Could you check a few things on this drawing? It's one solid part, dimensions in mm from its lowest x, y, z. A direction names the side the tool comes from. Give positions to 0.01 mm unless a question says otherwise; leave off trailing zeros. Loops run counter-clockwise (first coordinate to the right, second up) from the corner with the lowest first, then second, coordinate; pieces in that order, holes last. Notation, with made-up numbers: (66, 15.5) - (100, 15.5) arc R22 cw to (100, 41.5) - close; hole circle Ø1 at (-5, -11). An arc over 180 degrees is marked (long way). Return JSON: item names as keys, results as strings. Group by question number.
(1) I need wall thicknesses on probe 1 along X at (y, z) = (37.5, 27.5); probe 2 along Y at (x, z) = (89, 44.5); probe 3 along Z at (x, y) = (56, 85). Which ranges of each line are inside material? Lowest first, please. Write a range as [from, to].
(2) If we section it at D-D (y = 59): Please give me the cut outline in (x, z).
(3) If we section it at A-A (x = 30): Please give me the cut outline in (y, z).
(4) If we section it at B-B (y = 24): Please give me the cut outline in (x, z).
(5) If we section it at C-C (z = 30): Please give me the cut outline in (x, y), then the cut area to 3 significant figures.
(6) On a 3-axis mill with a long thin cutter (end or side, diameter ignored), from which of +Z, -Z, +X, -X, +Y, -Y can I reach the whole of each face in a straight line? I mean the marked faces 1 and 2. Say none if no direction works.
(7) For P1, Ø6, axis at x = 45.5, y = 11, coming from the -Z side; P2, Ø1.8, axis at x = 2.5, z = 9, coming from the +Y side; P3, Ø3, axis at x = 1, z = 16.5, coming from the -Y side, each with a flat end and sliding along its axis, tell me the tip position at first contact or that it passes through.
(8) If we mould it in two halves opening along X, with no side actions, what happens to the marked faces 3, 4 and 5? For each: released by +X, released by -X, zero draft, split by the parting line, or undercut.
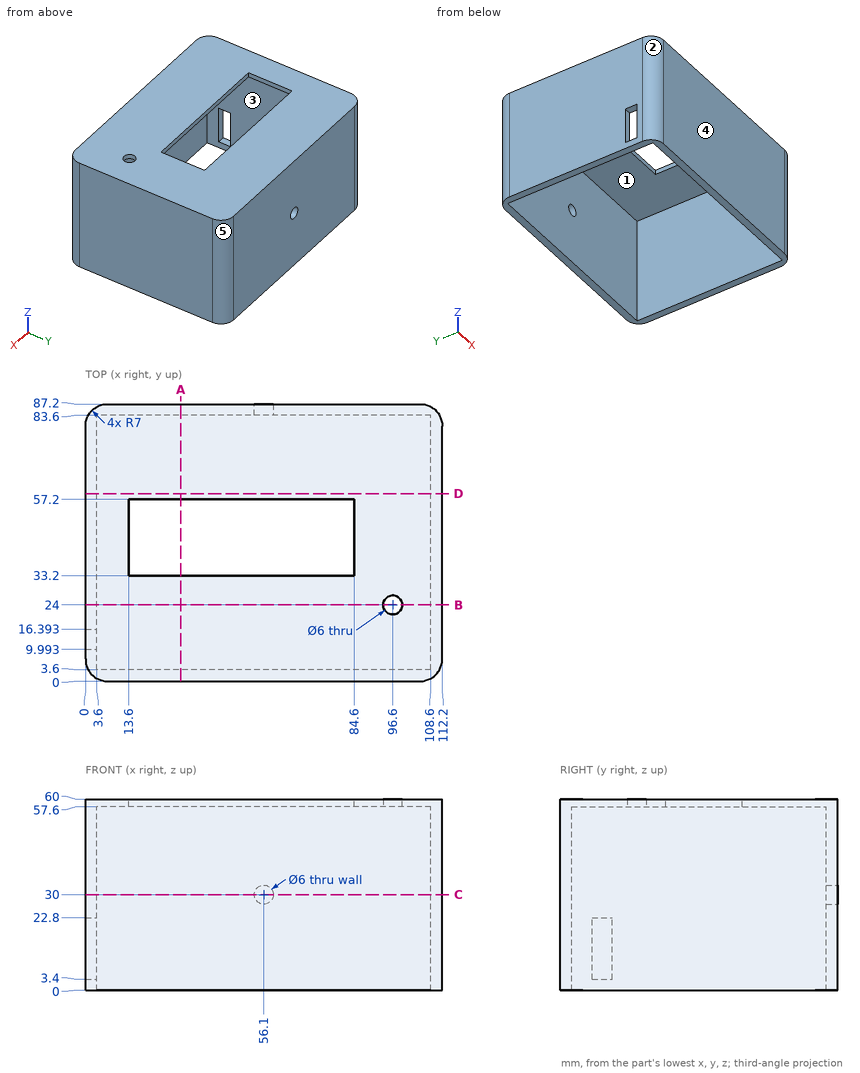
Values:
{
 "1": {"probe 1": "[0, 3.6], [108.6, 112.2]", "probe 2": "[0, 3.6], [83.6, 87.2]", "probe 3": "[0, 27], [33, 60]"},
 "2": {"outline": "(0, 0) - (3.6, 0) - (3.6, 57.6) - (108.6, 57.6) - (108.6, 0) - (112.2, 0) - (112.2, 60) - (0, 60) - close"},
 "3": {"outline": "(0, 0) - (3.6, 0) - (3.6, 57.6) - (33.2, 57.6) - (33.2, 60) - (0, 60) - close; (57.2, 57.6) - (83.6, 57.6) - (83.6, 0) - (87.2, 0) - (87.2, 60) - (57.2, 60) - close"},
 "4": {"outline": "(0, 0) - (3.6, 0) - (3.6, 57.6) - (93.6, 57.6) - (93.6, 60) - (0, 60) - close; (99.6, 57.6) - (108.6, 57.6) - (108.6, 0) - (112.2, 0) - (112.2, 60) - (99.6, 60) - close"},
 "5": {"outline": "(0, 7) arc R7 ccw to (7, 0) - (105.2, 0) arc R7 ccw to (112.2, 7) - (112.2, 80.2) arc R7 ccw to (105.2, 87.2) - (59.1, 87.2) - (59.1, 83.6) - (108.6, 83.6) - (108.6, 3.6) - (3.6, 3.6) - (3.6, 83.6) - (53.1, 83.6) - (53.1, 87.2) - (7, 87.2) arc R7 ccw to (0, 80.2) - close", "area": "1,320 mm2"},
 "6": {"face 1": "-Z", "face 2": "+Z, -Z, -X, -Y"},
 "7": {"P1": "z = 57.6", "P2": "y = 86.2", "P3": "y = 1.64"},
 "8": {"face 3": "undercut", "face 4": "zero draft", "face 5": "released by +X"}
}
